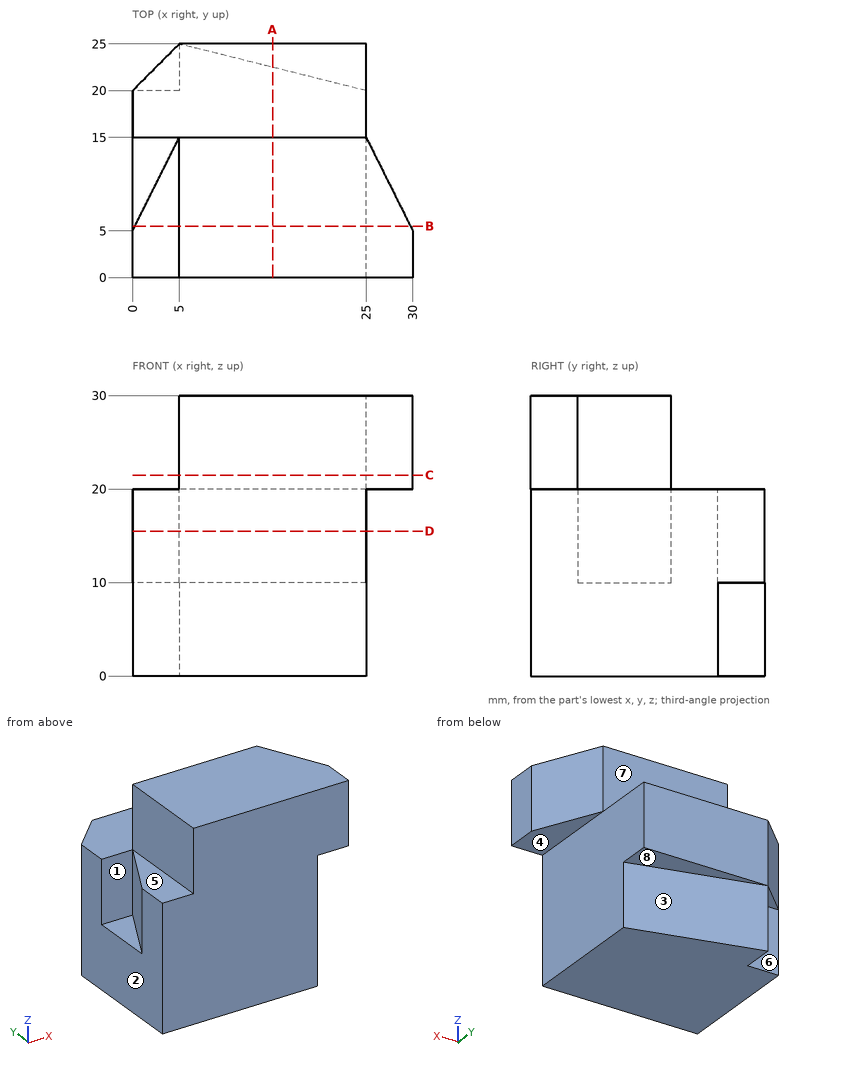
Job drawing, mm, ordinate dimensions from the low corner. One solid piece. A direction names the side the tool comes from. Round coordinates to 2 decimals unless told otherwise and drop trailing zeros. Write each loop counter-clockwise with the first axis right and the second up, starting at its lowest first coordinate (ties: lowest second). Pieces come first, ordered by that corner, then holes. Notation, with made-up numbers: (39, 23) -> (78, 23) arc R8 ccw to (78, 31) -> close; hole circle Ø4 at (-33.75, 55.5). An arc over 180 degrees is marked (long way). Answer as CSV lines item,"result".
1. Pin check, flat tips, straight feed: pin 1 Ø1.5 at (x, y) = (16.5, 23.5) entering from -Z; pin 2 Ø1.5 at (y, z) = (14.5, 22.5) entering from -X; pin 3 Ø6 at (x, z) = (26, 25) entering from +Y. Stop position of each tip, or through.
Resolved:
pin 1,"z = 10"
pin 2,"x = 5"
pin 3,"y = 15"
2. Drill centre lines: line 1 (Y direction, x = 8.75, z = 25.5); line 2 (Z direction, x = 1.5, y = 18); line 3 (X direction, y = 3, z = 24.5). Where is each one in solid material? Low to high.
Resolved:
line 1,"0 to 15"
line 2,"0 to 20"
line 3,"5 to 30"
3. Slice it at D-D, the plane z = 15.5. List the corners of the cut face in (x, y), plus the area to 4 significant figures.
Resolved:
outline,"(0, 0) -> (25, 0) -> (25, 25) -> (5, 25) -> (0, 20) -> (0, 15) -> (5, 15) -> (0, 5) -> close"
area,"587.5 mm²"
4. Slice it at C-C, the plane z = 21.5. List the corners of the cut face in (x, y), plus the area to 3 significant figures.
Resolved:
outline,"(5, 0) -> (30, 0) -> (30, 5) -> (25, 15) -> (5, 15) -> close"
area,"350 mm²"
5. Mould opens along Y. For the marked faces 1, 2 and 3 say: +Y half, -Y half, draft (parallel to the pull), parting line (faces both ways), or undercut.
Resolved:
face 1,"undercut"
face 2,"draft"
face 3,"+Y half"
6. Tool access for the marked faces 4, 5, 6, 7 and 8: list every direction of +Z, -Z, +X, -X, +Y, -Y with a clear straight run to the whole face (end or side of a thin tool).
Resolved:
face 4,"-Z, +X, +Y, -Y"
face 5,"+Z, -X, +Y, -Y"
face 6,"-Z, -X, +Y"
face 7,"+Z, +X, -X, +Y"
face 8,"-Z, +X, +Y"
7. Slice it at B-B, the plane y = 5.5. List the corners of the cut face in (x, z), plus the area to 3 significant figures.
Resolved:
outline,"(0, 0) -> (25, 0) -> (25, 20) -> (29.75, 20) -> (29.75, 30) -> (5, 30) -> (5, 20) -> (0.25, 20) -> (0.25, 10) -> (0, 10) -> close"
area,"745 mm²"
8. Slice it at A-A, the plane x = 15. List the corners of the cut face in (y, z), plus the area to 3 significant figures.
Resolved:
outline,"(0, 0) -> (22.5, 0) -> (22.5, 10) -> (25, 10) -> (25, 20) -> (15, 20) -> (15, 30) -> (0, 30) -> close"
area,"625 mm²"
